Answer from the drawing. Dimensions are ordinates in mm from the lowest x, y and z of the part. Coordinates: 2 decimals unless noted, no trailing zeros. Order: outer loops, then holes, each group sorted by start corner. A loop starts at its lowest first (then second) coordinate and runs counter-clockwise, first axis right, second up. Notation, with made-up numbers: (56.25, 23) -> (107.25, 23) arc R24 ccw to (107.25, 56) -> close; hole circle Ø2 at (53.25, -22.75). An arc over 180 degrees is marked (long way). Use CSV: the item, a comma, the result in double quotes.
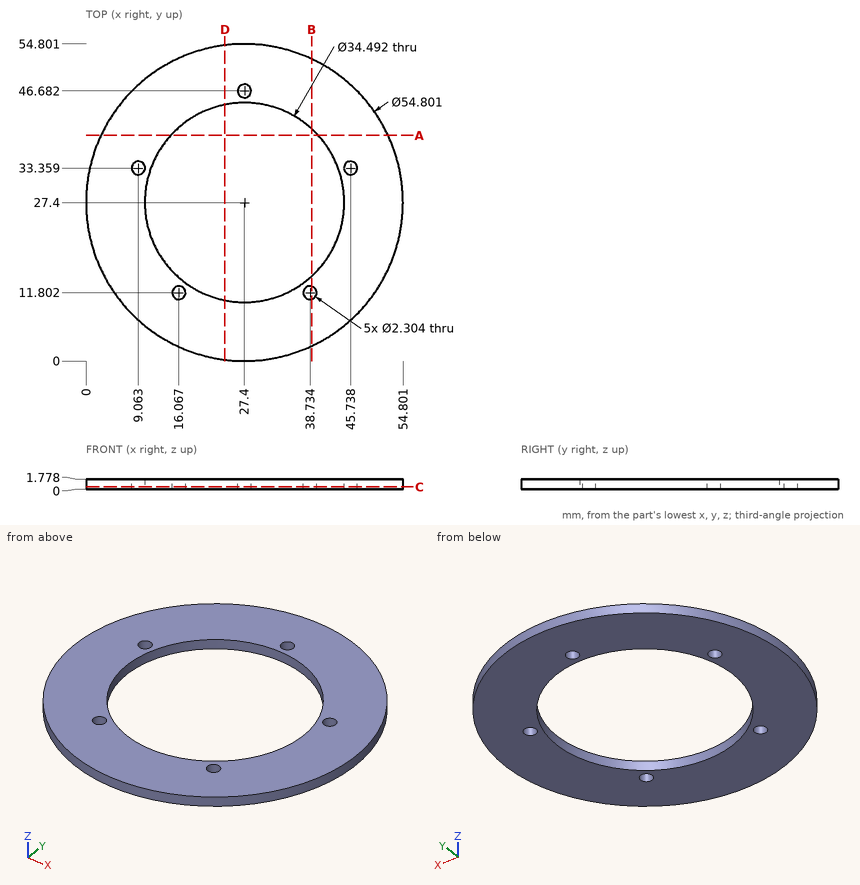
Item 1: Find section D-D, the plane x = 24. Give the vertices of the cut face in (y, z).
Return value:
outline,"(0.21, 0) -> (10.49, 0) -> (10.49, 1.78) -> (0.21, 1.78) -> close; (44.31, 0) -> (54.59, 0) -> (54.59, 1.78) -> (44.31, 1.78) -> close"
Item 2: Find section B-B, the plane x = 39. Give the vertices of the cut face in (y, z) (1 decimal).
Return value:
outline,"(2.6, 0) -> (10.7, 0) -> (10.7, 1.8) -> (2.6, 1.8) -> close; (12.9, 0) -> (14.6, 0) -> (14.6, 1.8) -> (12.9, 1.8) -> close; (40.2, 0) -> (52.2, 0) -> (52.2, 1.8) -> (40.2, 1.8) -> close"
Item 3: Find section A-A, the plane y = 39. Give the vertices of the cut face in (x, z) (1 decimal).
Return value:
outline,"(2.6, 0) -> (14.6, 0) -> (14.6, 1.8) -> (2.6, 1.8) -> close; (40.2, 0) -> (52.2, 0) -> (52.2, 1.8) -> (40.2, 1.8) -> close"
Item 4: Find section C-C, the plane z = 0.4. Give the vertices of the cut face in (x, y) (1 decimal).
Return value:
outline,"circle Ø54.8 at (27.4, 27.4); hole circle Ø2.3 at (9.1, 33.4); hole circle Ø34.5 at (27.4, 27.4); hole circle Ø2.3 at (16.1, 11.8); hole circle Ø2.3 at (27.4, 46.7); hole circle Ø2.3 at (38.7, 11.8); hole circle Ø2.3 at (45.7, 33.4)"
Item 5: Each of these flat-tipped pins is pushed along its axis until it touches: P1, Ø1, axis at y = 48, z = 1.5, coming from the +X side; P2, Ø1, axis at x = 9, z = 1, coming from the +Y side (1 decimal). Where does it stop, or does it pass through?
Return value:
P1,"stops at x = 46.02"
P2,"stops at y = 48.1"
Item 6: Straight lines are drawn through the part: line 1 along Y through (x, z) = (39.5, 0.65) (1 decimal); line 2 along X through (y, z) = (27, 0.15); line 3 along Y through (x, z) = (16.5, 1.05) (1 decimal). For each, find the intervals that lie inside material, in ascending order.
Return value:
line 1,"y = 2.8 to 10.9, 12.7 to 15.1, 39.7 to 52"
line 2,"x = 0 to 10.16, 44.64 to 54.8"
line 3,"y = 2.3 to 10.7, 12.9 to 14, 40.8 to 52.5"
